Read the model definition and answer for the solid it produces. Units are mm, in the model's axes. Give positions to 0.01 mm unless a question says otherwise; leave off trailing zeros. Order: outer loops, then holes, each group sorted by start corner. A loop starts at its lowest first (then second) coordinate and runs counter-clockwise, first axis right, second up. Notation, with made-up numbers: (13, -30.75) -> (23, -30.75) arc R11 ccw to (23, -12.75) -> close; hole circle Ø11 at (36.25, 50.25). An arc over 180 degrees is marked (long way). One line per question, with ' | ' between items. Start each with the question number.
```python
from build123d import *

# Parameters (mm, degrees)
SZKIC1_R                    = 8
SZKIC1_R_2                  = 4
DODANIE_WYCI_GNI_CIE1_DEPTH = 120
SZKIC2_R                    = 5
WYTNIJ_WYCI_GNI_CIE1_DEPTH  = 40
WYTNIJ_WYCI_GNI_CIE2_START  = -30
SZKIC3_R                    = 5
WYTNIJ_WYCI_GNI_CIE2_DEPTH  = 30


with BuildPart() as part:
    # Szkic1 → Dodanie-wyciągnięcie1 (new, symmetric)
    with BuildSketch(Plane.XY):
        Circle(SZKIC1_R)
        Circle(SZKIC1_R_2, mode=Mode.SUBTRACT)
    extrude(amount=DODANIE_WYCI_GNI_CIE1_DEPTH, both=True)

    # Szkic2 → Wytnij-wyciągnięcie1 (cut)
    with BuildSketch(Plane.XY.offset(120)):
        Circle(SZKIC2_R)
    extrude(amount=-WYTNIJ_WYCI_GNI_CIE1_DEPTH, mode=Mode.SUBTRACT)

    # Szkic3 → Wytnij-wyciągnięcie2 (cut)
    with BuildSketch(Plane(origin=(0, 0, -120), x_dir=(-1, 0, 0), z_dir=(0, 0, -1)).offset(WYTNIJ_WYCI_GNI_CIE2_START)):
        with Locations(Location((0, 0, 0), (0, 0, 180))):
            Circle(SZKIC3_R)
    extrude(amount=WYTNIJ_WYCI_GNI_CIE2_DEPTH, mode=Mode.SUBTRACT)


solid = part.part
```
Q1. Given P1, Ø3, axis at y = 2, z = 93.5, coming from the +X side; P2, Ø1, axis at y = -4, z = 26, coming from the +X side; P3, Ø3, axis at x = -2, y = 1, coming from the +Z side; P4, Ø4, axis at x = -2.5, z = 38, coming from the +Y side, each flat-ended and moving along its own axis, determine where each tip first touches the part or whether it passes through.
Q2. Determine the mould class of faces 1 (the flat face through (5.2, 0.1, 120)), 2 (the cylindrical face through (-5, 0, -105)), 3 (the cylindrical face through (-1.73, -7.81, 1.68)), 4 (the cylindrical face through (-1.08, -4.88, 100.28)) for opening direction Y: pulls with the +Y half, pulls with the -Y half, needs draft (parallel to the pull), parting line crosses it, or undercut.
Q3. A cutting plane is placed at A-A, the plane x = 0. Determine the outline of the cut face in (y, z).
Q4. Find the intervals of material crossed by line 1 (Y direction, x = 0, z = -100.5); line 2 (Z direction, x = 4, y = -0.75); line 3 (Y direction, x = 0.75, z = -16.5), in increasing order.
Q5. A cutting plane is placed at D-D, the plane z = -69.5. Determine the outline of the cut face in (x, y).
Q6. A cutting plane is placed at C-C, the plane z = -99.5. Determine the outline of the cut face in (x, y), then the cut area to 3 significant figures.
Geometry results:
1) P1: x = 7.98 | P2: x = 7.19 | P3: through | P4: y = 7.98
2) face 1: needs draft | face 2: undercut | face 3: parting line crosses it | face 4: undercut
3) outline: (-8, -120) -> (-5, -120) -> (-5, -90) -> (-4, -90) -> (-4, 80) -> (-5, 80) -> (-5, 120) -> (-8, 120) -> close; (4, -90) -> (5, -90) -> (5, -120) -> (8, -120) -> (8, 120) -> (5, 120) -> (5, 80) -> (4, 80) -> close
4) line 1: -8 to -5, 5 to 8 | line 2: -90 to 80 | line 3: -7.96 to -3.93, 3.93 to 7.96
5) outline: circle Ø16 at (0, 0); hole circle Ø8 at (0, 0)
6) outline: circle Ø16 at (0, 0); hole circle Ø10 at (0, 0) | area: 123 mm²
